Design review of the part built by this model. Coordinates are the model's own, in mm. Face numbers are marked on the shaded views. A direction names the side the tool comes from. Give positions to 0.01 mm unless a question says otherwise; leave off trailing zeros. Write each loop counter-clockwise with the first axis right and the second up, starting at its lowest first coordinate (ties: lowest second). Pieces come first, ordered by that corner, then holes. Notation, with made-up numbers: (-38.75, -7.5) -> (-11.75, -7.5) arc R12 cw to (-11.75, 14.5) -> close; hole circle Ø4 at (-12.75, 63.25). An arc over 180 degrees is marked (long way). Answer as a JSON object with one key per item and string values.
```python
from build123d import *

# Parameters (mm, degrees)
SKETCH1_W           = 190
SKETCH1_H           = 285
BOSS_EXTRUDE1_DEPTH = 30
CUT_EXTRUDE1_DEPTH  = 32
SKETCH4_R           = 1.5
CUT_EXTRUDE2_DEPTH  = 40
CUT_EXTRUDE3_START  = 45
CUT_EXTRUDE3_DEPTH  = 51
CUT_EXTRUDE4_START  = -45
CUT_EXTRUDE4_DEPTH  = 51
CHAMFER1_SIZE       = 13
SKETCH6_R           = 1.5
CUT_EXTRUDE5_DEPTH  = 5


with BuildPart() as part:
    # Sketch1 → Boss-Extrude1 (new body)
    with BuildSketch(Plane(origin=(0, 0, 0), x_dir=(1, 0, 0), z_dir=(0, 1, 0))):
        Rectangle(SKETCH1_W, SKETCH1_H)
    extrude(amount=BOSS_EXTRUDE1_DEPTH)

    # Sketch3 → Cut-Extrude1 (cut)
    with BuildSketch(Plane(origin=(0, 0, -142.5), x_dir=(-1, 0, 0), z_dir=(0, 0, -1))):
        Polygon((-37.5, 30), (37.5, 30), (42.5, 0), (-42.5, 0), align=None)
    extrude(amount=-CUT_EXTRUDE1_DEPTH, mode=Mode.SUBTRACT)

    # Sketch4 → Cut-Extrude2 (cut)
    with BuildSketch(Plane(origin=(0, 0, -110.5), x_dir=(-1, 0, 0), z_dir=(0, 0, -1))):
        with Locations((-25, 14)):
            Circle(SKETCH4_R)
        with Locations(Location((25, 14, 0), (0, 0, 180))):  # turned: the seam where the file's is
            Circle(SKETCH4_R)
    extrude(amount=-CUT_EXTRUDE2_DEPTH, mode=Mode.SUBTRACT)

    # Sketch5 → Cut-Extrude3 (cut, through all)
    with BuildSketch(Plane(origin=(0, 0, 0), x_dir=(0, 0, -1), z_dir=(1, 0, 0)).offset(CUT_EXTRUDE3_START)):
        Polygon((129.5, 30), (142.5, 17), (142.5, 30), align=None)
    extrude(amount=CUT_EXTRUDE3_DEPTH, mode=Mode.SUBTRACT)

    # Sketch5_2 → Cut-Extrude4 (cut, through all)
    with BuildSketch(Plane(origin=(0, 0, 0), x_dir=(0, 0, -1), z_dir=(1, 0, 0)).offset(CUT_EXTRUDE4_START)):
        Polygon((129.5, 30), (142.5, 17), (142.5, 30), align=None)
    extrude(amount=-CUT_EXTRUDE4_DEPTH, mode=Mode.SUBTRACT)

    # Chamfer1
    chamfer1_edges = [part.edges().sort_by_distance(p)[0] for p in [
        (-95, 30, 6.5),
        (0, 30, 142.5),
        (95, 30, 6.5),
    ]]
    chamfer(chamfer1_edges, length=CHAMFER1_SIZE)

    # Sketch6 → Cut-Extrude5 (cut)
    with BuildSketch(Plane.XZ):
        with Locations(Location((-75, 122.5, 0), (0, 0, 270))):  # turned: the seam where the file's is
            Circle(SKETCH6_R)
        with Locations(Location((75, 122.5, 0), (0, 0, 270))):  # turned: the seam where the file's is
            Circle(SKETCH6_R)
        with Locations(Location((-75, -122.5, 0), (0, 0, 270))):  # turned: the seam where the file's is
            Circle(SKETCH6_R)
        with Locations(Location((75, -122.5, 0), (0, 0, 270))):  # turned: the seam where the file's is
            Circle(SKETCH6_R)
    extrude(amount=-CUT_EXTRUDE5_DEPTH, mode=Mode.SUBTRACT)


solid = part.part
```
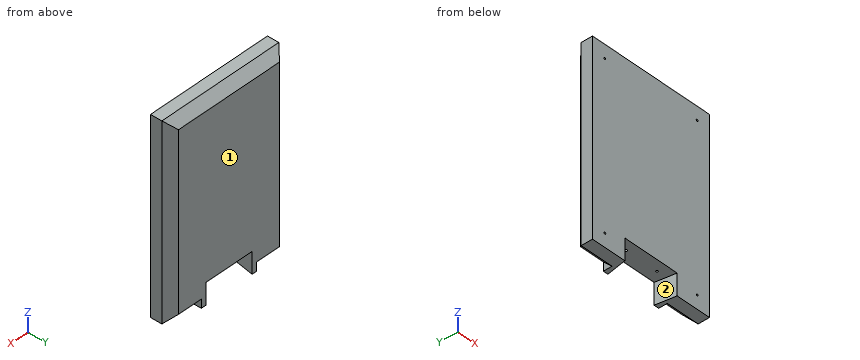
(1) For line 1 along X through (y, z) = (3.4, 122.5); line 2 along Z through (x, y) = (-75, 3.55); line 3 along Y through (x, z) = (-25, -101), list the stretches that pass through material, from the lowest coordinate up.
Here are the results:
{"line 1": "x = -95 to -76.5, -73.5 to 73.5, 76.5 to 95", "line 2": "z = -142.5 to -124, -121 to 121, 124 to 142.5", "line 3": "y = 0 to 12.5, 15.5 to 30"}
(2) We need section B-B, the plane x = 57. State the section outline as (y, z) points.
Here are the results:
{"outline": "(0, -142.5) -> (17, -142.5) -> (30, -129.5) -> (30, 129.5) -> (17, 142.5) -> (0, 142.5) -> close"}
(3) Clearance check with flat-ended pins moving along their axes: pin 1 (4 mm diameter, centred on y = 25.5, z = 90, fed in from -X); pin 2 (3.5 mm diameter, centred on x = 25.5, y = 14.5, fed in from -Z); pin 3 (2.5 mm diameter, centred on x = -75, z = 122.5, fed in from -Y). State where each tip first meets the part, or that it passes through.
Here are the results:
{"pin 1": "stops at x = -88.5", "pin 2": "stops at z = -110.5", "pin 3": "stops at y = 5"}
(4) We need section C-C, the plane z = 36.5. State the section outline as (x, y) points, then the cut area to 3 significant figures.
Here are the results:
{"outline": "(-95, 0) -> (95, 0) -> (95, 17) -> (82, 30) -> (-82, 30) -> (-95, 17) -> close", "area": "5,530 mm²"}
(5) We need section A-A, the plane y = 22.5. State the section outline as (x, z) points, then the cut area to 3 significant figures.
Here are the results:
{"outline": "(-89.5, -137) -> (-45, -137) -> (-45, -142.5) -> (-38.75, -142.5) -> (-38.75, -110.5) -> (38.75, -110.5) -> (38.75, -142.5) -> (45, -142.5) -> (45, -137) -> (89.5, -137) -> (89.5, 137) -> (-89.5, 137) -> close", "area": "47,100 mm²"}
(6) For the marked faces 1 and 2, list the 3-axis set-ups (+Z, -Z, +X, -X, +Y, -Y) from which the entire face can be reached by the end or side of a thin tool; tool diameter is ignored.
Here are the results:
{"face 1": "+Z, -Z, +X, -X, +Y", "face 2": "-Z, -Y"}
(7) We need section D-D, the plane x = 33. State the section outline as (y, z) points, then the cut area to 3 significant figures.
Here are the results:
{"outline": "(0, -110.5) -> (30, -110.5) -> (30, 129.5) -> (17, 142.5) -> (0, 142.5) -> close", "area": "7,510 mm²"}
